CAD build for the part. Positions are in the model's coordinates, mm. Face numbers are marked on the shaded views. A direction names the side the tool comes from. Give positions to 0.01 mm unless a question says otherwise; leave off trailing zeros.
Item 1: Two-plate mould, pull along Z, no slides. Class the marked faces 3, 4 and 5: released by +Z, released by -Z, zero draft, split by the parting line, or undercut.
Item 2: Flat gauge pins, fed straight in: P1, Ø6, axis at y = -27.5, z = 70.5, coming from the -X side; P2, Ø4, axis at x = -30.5, y = 2, coming from the -Z side; P3, Ø10, axis at y = -30, z = 42, coming from the +X side. Where does each tip first touch, or does it go through?
Item 3: Which spindle directions (+Z, -Z, +X, -X, +Y, -Y) get a long thin tool onto all of the face, cutting with end or side? Do the marked faces 1 and 2. Say none if no direction does.
Item 4: Wall check: L1, parallel to X at y = 33, z = 88; L2, parallel to Z at x = -46.5, y = 31; L3, parallel to X at y = -19, z = 137.5. Give the ranges that are in metal, low to high.
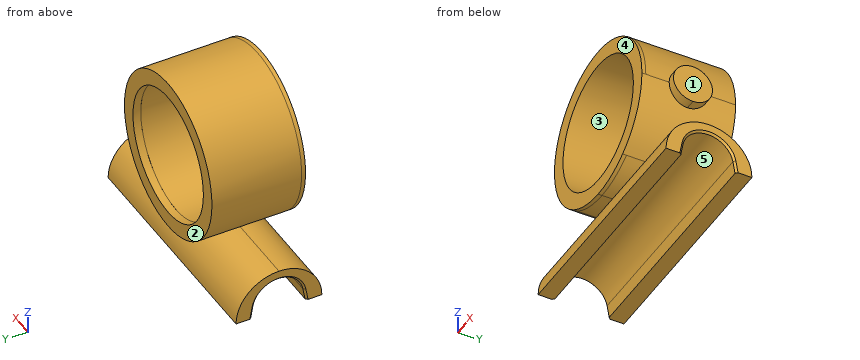
```python
from build123d import *
from build123d import SkipClean  # not in build123d's __all__

# Parameters (mm, degrees)
F0_W            = 190.5
F0_H            = 69.85
F1_DEPTH        = 34.925
F4_DEPTH        = 190.5
F5_DEPTH        = 73.025
F6_DEPTH        = 3.175
F9_DEPTH        = 190.5010001
F10_SIZE2       = 1.5875
F10_SIZE        = 1.5875
F14_DEPTH       = 36.64824
F16_DEPTH       = 83.54939
F17_D           = 104.775
F17_CBORE_D     = 104.8004
F17_CBORE_DEPTH = 6.35


with BuildPart() as f1:
    # F0 (on Top) → F1 (new body)
    with BuildSketch(Plane.XY):
        Rectangle(F0_W, F0_H)
    extrude(amount=F1_DEPTH)

    # F2 (on face) → F4 (cut)
    with BuildSketch(Plane.YZ.offset(95.25)):
        with BuildLine():
            Line((-34.925, 34.925), (-34.925, 0))
            ThreePointArc((-34.925, 0), (-24.6957043451, 24.6957043208), (-3.45e-08, 34.925))
            Line((-3.45e-08, 34.925), (-34.925, 34.925))
        make_face()
        with BuildLine():
            ThreePointArc((-3.45e-08, 34.925), (24.6957043208, 24.6957043451), (34.925, 0))
            Line((34.925, 0), (34.925, 34.925))
            Line((34.925, 34.925), (-3.45e-08, 34.925))
        make_face()
    extrude(amount=-F4_DEPTH, mode=Mode.SUBTRACT)

    # F3 (on face) → F5 (join)
    with BuildSketch(Plane.XZ.offset(34.925)):
        with BuildLine():
            Line((-36.3741945787, 34.925), (0, 34.925))
            Line((0, 34.925), (36.3741945787, 34.925))
            ThreePointArc((36.3741945787, 34.925), (57.462544522, 58.3314110024), (65.0875, 88.9))
            ThreePointArc((65.0875, 88.9), (-30.5685889976, 146.362544522), (-36.3741945787, 34.925))
        make_face()
        with BuildLine():
            Line((0, 34.925), (0, 23.8125))
            ThreePointArc((0, 23.8125), (19.0168983243, 26.6525885327), (36.3741945787, 34.925))
            Line((36.3741945787, 34.925), (0, 34.925))
        make_face()
        with BuildLine():
            ThreePointArc((-36.3741945787, 34.925), (-19.0168983243, 26.6525885327), (0, 23.8125))
            Line((0, 23.8125), (0, 34.925))
            Line((0, 34.925), (-36.3741945787, 34.925))
        make_face()
    with SkipClean():  # cleaning this boolean's faces spoils the solid; the shape is the same uncleaned
        extrude(amount=-F5_DEPTH)

    # F6 (add): a face of the model
    f6_faces = [f1.faces().sort_by_distance(p)[0] for p in [
        (0, -34.925, 88.9),
    ]]
    with SkipClean():  # cleaning this boolean's faces spoils the solid; the shape is the same uncleaned
        extrude(f6_faces, amount=F6_DEPTH)

    # F8 (on face) → F9 (cut, through all)
    with BuildSketch(Plane.YZ.offset(95.25)):
        with BuildLine():
            Line((22.0755430303, 0), (20.3239700028, 9.9336642666))
            ThreePointArc((20.3239700028, 9.9336642666), (0, 26.9875), (-20.3239700028, 9.9336642666))
            Line((-20.3239700028, 9.9336642666), (-22.0755430303, 0))
            Line((-22.0755430303, 0), (0, 0))
            Line((0, 0), (22.0755430303, 0))
        make_face()
    with SkipClean():  # cleaning this boolean's faces spoils the solid; the shape is the same uncleaned
        extrude(amount=-F9_DEPTH, mode=Mode.SUBTRACT)

    # F10
    f10_edges = [f1.edges().sort_by_distance(p)[0] for p in [
        (95.25, 0, 26.9875),
        (95.25, 21.199757, 4.966832),
        (95.25, -21.199757, 4.966832),
        (-95.25, 0, 26.9875),
        (-95.25, -21.199757, 4.966832),
        (-95.25, 21.199757, 4.966832),
    ]]
    chamfer(f10_edges, length=F10_SIZE, length2=F10_SIZE2)

    # F13 (on face) → F14 (join)
    with BuildSketch(Plane.YZ.offset(95.25)):
        with BuildLine():
            ThreePointArc((15.875, 88.9), (-11.2253201513, 100.1253201513), (0, 73.025))
            ThreePointArc((0, 73.025), (11.2253201513, 77.6746798487), (15.875, 88.9))
        make_face()
    with SkipClean():  # cleaning this boolean's faces spoils the solid; the shape is the same uncleaned
        extrude(amount=-F14_DEPTH)

    # F15 (on face) → F16 (cut)
    with BuildSketch(Plane.XZ.offset(38.1)):
        Polygon((71.4375, 107.923515141), (71.4375, 88.9), (71.4375, 69.2154169083), (71.4375, 68.7513798475), (104.9063950777, 68.7513798475), (104.9063950777, 107.923515141), align=None)
    with SkipClean():  # cleaning this boolean's faces spoils the solid; the shape is the same uncleaned
        extrude(amount=-F16_DEPTH, mode=Mode.SUBTRACT)

    # F17 (through all)
    with Locations(Plane(origin=(0, 38.1, 0), x_dir=(-1, 0, 0), z_dir=(0, 1, 0))):
        with Locations((0, 88.9)):
            CounterBoreHole(F17_D / 2, F17_CBORE_D / 2, F17_CBORE_DEPTH)


solid = f1.part
```
The answers:
1. face 3: undercut
1. face 4: zero draft
1. face 5: released by -Z
2. P1: stops at x = -63.24
2. P2: stops at z = 26.6
2. P3: stops at x = 49.81
3. face 1: +Z, +X, +Y, -Y
3. face 2: +Z, -Z, +X, -X, +Y
4. L1: x = -65.08 to -52.39, 52.39 to 65.08
4. L2: z = 0 to 16.09, 43.36 to 64.77, 113.03 to 134.44
4. L3: x = -43.29 to -19.56, 19.56 to 43.29
